Geometry: final body of the model. Coordinates: model frame, mm. Face numbers are marked on the shaded views. A direction names the side the tool comes from. Round coordinates to 2 decimals unless told otherwise and drop trailing zeros. Order: outer loops, then holes, each group sorted by start corner. A loop starts at its lowest first (then second) coordinate and runs counter-clockwise, first axis right, second up. Notation, with made-up numbers: (-36, -2) -> (-31, -2) arc R32 ccw to (-31, 37) -> close; hole circle Ø1 at (55, -25.5). An arc over 180 degrees is marked (long way). Put each result on its own line as item: value.
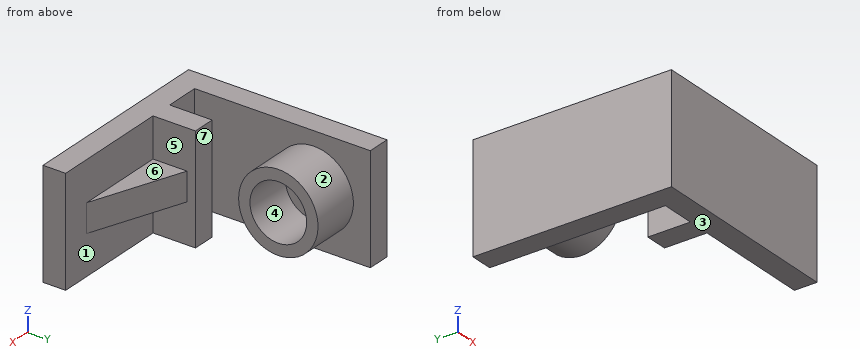
```python
from build123d import *

# Parameters (mm, degrees)
BOSS_EXTRUDE1_DEPTH = 38
RIB1_REACH          = 65.674
SKETCH2_WALL_W      = 163.52442716
SKETCH2_WALL_H      = 10
SKETCH3_R           = 14
SKETCH3_R_2         = 10
BOSS_EXTRUDE2_DEPTH = 17


with BuildPart() as part:
    # Sketch1 → Boss-Extrude1 (new body)
    with BuildSketch(Plane.XY):
        Polygon((-16.097560976, 39.829268293), (-24.097560976, 39.829268293), (-24.097560976, -30.170731707), (45.902439024, -30.170731707), (45.902439024, -22.170731707), (3.902439024, -22.170731707), (3.902439024, -7.170731707), (-4.097560976, -7.170731707), (-4.097560976, -22.170731707), (-16.097560976, -22.170731707), align=None)
    extrude(amount=BOSS_EXTRUDE1_DEPTH)

    # Sketch2 wall → Rib1 (add, up to next)
    with BuildSketch(Plane(origin=(19.902439024, -16.170731707, 19), x_dir=(0.936329177569, -0.351123441588, 0), z_dir=(0.351123441588, 0.936329177569, 0)), mode=Mode.PRIVATE) as rib1_sk1:
        Rectangle(SKETCH2_WALL_W, SKETCH2_WALL_H)
    rib1_tool1 = extrude(rib1_sk1.sketch, amount=-RIB1_REACH, mode=Mode.PRIVATE) - part.part
    add(rib1_tool1.solids().sort_by_distance((19.902439024, -16.170731707, 19))[0])

    # Sketch3 → Boss-Extrude2 (add)
    with BuildSketch(Plane(origin=(-16.097560976, 0, 0), x_dir=(0, 0, -1), z_dir=(1, 0, 0))):
        with Locations(Location((-19, 19.829268293, 0), (0, 0, 270))):
            Circle(SKETCH3_R)
        with Locations(Location((-19, 19.829268293, 0), (0, 0, 90))):
            Circle(SKETCH3_R_2, mode=Mode.SUBTRACT)
    extrude(amount=BOSS_EXTRUDE2_DEPTH)


solid = part.part
```
1. Cut plane A-A on x = -12. Return loops of the section in (y, z), and give its area (3 significant figures).
Ans:
outline: (-30.17, 0) -> (-22.17, 0) -> (-22.17, 38) -> (-30.17, 38) -> close; circle Ø28 at (19.83, 19); hole circle Ø20 at (19.83, 19)
area: 606 mm²
2. Set-up query: the marked faces 5, 6 and 7. Return all of +Z, -Z, +X, -X, +Y, -Y with unobstructed straight access to the full face (end or side cutting, diameter ignored); none if empty.
Ans:
face 5: +X, +Y
face 6: +Z, +X, +Y
face 7: +Z, -Z, +X
3. Cut plane B-B on z = 19. Return loops of the section in (x, y), and give its area (3 significant figures).
Ans:
outline: (-24.1, -30.17) -> (45.9, -30.17) -> (45.9, -22.17) -> (35.9, -22.17) -> (3.9, -10.17) -> (3.9, -7.17) -> (-4.1, -7.17) -> (-4.1, -22.17) -> (-16.1, -22.17) -> (-16.1, 5.83) -> (0.9, 5.83) -> (0.9, 9.83) -> (-16.1, 9.83) -> (-16.1, 29.83) -> (0.9, 29.83) -> (0.9, 33.83) -> (-16.1, 33.83) -> (-16.1, 39.83) -> (-24.1, 39.83) -> close
area: 1,500 mm²
4. Cut plane D-D on y = 13. Return loops of the section in (x, z), and give its area (3 significant figures).
Ans:
outline: (-24.1, 0) -> (-16.1, 0) -> (-16.1, 6.78) -> (0.9, 6.78) -> (0.9, 11.7) -> (-16.1, 11.7) -> (-16.1, 26.3) -> (0.9, 26.3) -> (0.9, 31.22) -> (-16.1, 31.22) -> (-16.1, 38) -> (-24.1, 38) -> close
area: 471 mm²
5. Contact query for flat-ended pins moving along their axis: P1, Ø6.5, axis at x = 0, z = 25.5, coming from the +Y side; P2, Ø4, axis at x = -0.5, z = 17.5, coming from the +Y side; P3, Ø8, axis at x = -16, y = -9, coming from the -Z side; P4, Ø14, axis at y = 21.5, z = 17, coming from the +X side. Output: stop coordinate, or through.
Ans:
P1: y = 33.45
P2: y = 33.83
P3: z = 0
P4: x = -16.1
6. Draft query along Y for the marked faces 1, 2, 3 and 4. Return one class per face: +Y half, -Y half, draft (parallel to the pull), parting line (faces both ways), or undercut.
Ans:
face 1: +Y half
face 2: undercut
face 3: draft
face 4: undercut
7. Material intervals for probe 1 along Y at (x, z) = (-11, 23.5); probe 2 along X at (y, z) = (-7.5, 3.5); probe 3 along X at (y, z) = (10.5, 16.5), sorted ascending.
Ans:
probe 1: -30.17 to -22.17, 6.57 to 10.9, 28.76 to 33.09
probe 2: -24.1 to -16.1, -4.1 to 3.9
probe 3: -24.1 to -16.1
8. Cut plane C-C on x = 0. Return loops of the section in (y, z).
Ans:
outline: (-30.17, 0) -> (-7.17, 0) -> (-7.17, 38) -> (-30.17, 38) -> close; circle Ø28 at (19.83, 19); hole circle Ø20 at (19.83, 19)
